from build123d import *

# Parameters (mm, degrees)
BOSS_EXTRUDE1_DEPTH = 70
FILLET1_R           = 10
SKETCH4_R           = 44.565838739
SKETCH4_R_2         = 21.950927137
CUT_EXTRUDE18_DEPTH = 5
SHELL2_START        = 10
SHELL2_DEPTH        = 50
SHELL2_START_2      = -77.141831355
SHELL2_2_OUTLINE_R  = 11.950927137
SHELL2_2_DEPTH      = 25
SKETCH2_R           = 10
CUT_EXTRUDE19_DEPTH = 30
SKETCH10_R          = 7.386058148
CUT_EXTRUDE22_DEPTH = 33
CUT_EXTRUDE23_DEPTH = 131.776604246
SKETCH16_W          = 25
SKETCH16_H          = 5
CUT_EXTRUDE25_DEPTH = 16.122153735
SKETCH17_W          = 25
SKETCH17_H          = 5
CUT_EXTRUDE26_DEPTH = 16.122153735


with BuildPart() as part:
    # Sketch1 → Boss-Extrude1 (new body)
    with BuildSketch(Plane.XY):
        Polygon((-85.15522278, 32.602281584), (85.31682344, 32.602281584), (107.858168645, -0.126017705), (84.012402994, -31.916476628), (-83.600577489, -31.916476628), (-92.141831355, -19.515233034), (-92.141831355, 19.263197625), align=None)
    extrude(amount=BOSS_EXTRUDE1_DEPTH)

    # Fillet1
    fillet1_edges = [part.edges().sort_by_distance(p)[0] for p in [
        (-88.648527067, 25.932739604, 0),
        (-85.15522278, 32.602281584, 35),
        (85.31682344, 32.602281584, 35),
        (107.858168645, -0.126017705, 35),
        (-87.871204422, -25.715854831, 70),
        (84.012402994, -31.916476628, 35),
        (-83.600577489, -31.916476628, 35),
        (-92.141831355, -19.515233034, 35),
        (-92.141831355, 19.263197625, 35),
        (0.205912752, -31.916476628, 70),
        (95.93528582, -16.021247166, 70),
        (96.587496042, 16.23813194, 70),
        (0.08080033, 32.602281584, 70),
        (-88.648527067, 25.932739604, 70),
        (0.08080033, 32.602281584, 0),
        (96.587496042, 16.23813194, 0),
        (95.93528582, -16.021247166, 0),
        (0.205912752, -31.916476628, 0),
        (-92.141831355, -0.126017705, 70),
        (-87.871204422, -25.715854831, 0),
        (-92.141831355, -0.126017705, 0),
    ]]
    fillet(fillet1_edges, radius=FILLET1_R)

    # Sketch4 → Cut-Extrude18 (cut)
    with BuildSketch(Plane(origin=(-62.141831355, 0, 0), x_dir=(0, 0, -1), z_dir=(1, 0, 0))):
        with Locations((-35, -0.126017705)):
            Circle(SKETCH4_R)
        with Locations(Location((-35, -0.126017705, 0), (0, 0, 90))):
            Circle(SKETCH4_R_2, mode=Mode.SUBTRACT)
    extrude(amount=-CUT_EXTRUDE18_DEPTH, mode=Mode.SUBTRACT)

    # Shell2: read off the stored shape, not the designer's step
    # Shell2 outline → Shell2 (cut)
    with BuildSketch(Plane.XY.offset(SHELL2_START)):
        Polygon((-78.345650785, -21.916476628), (-77.141831355, -21.916476628), (-77.141831355, 22.602281584), (-79.104276607, 22.602281584), (-82.141831355, 16.80287299), (-82.141831355, -16.404714454), align=None)
        Polygon((-52.141831355, -21.916476628), (79.012770562, -21.916476628), (95.544357754, 0.122939143), (80.061896735, 22.602281584), (-52.141831355, 22.602281584), align=None)
    extrude(amount=SHELL2_DEPTH, mode=Mode.SUBTRACT)

    # Shell2 2 outline → Shell2 2 (cut)
    with BuildSketch(Plane.YZ.offset(SHELL2_START_2)):
        with Locations((-0.126017705, 35)):
            Circle(SHELL2_2_OUTLINE_R)
    extrude(amount=SHELL2_2_DEPTH, mode=Mode.SUBTRACT)

    # Sketch2 → Cut-Extrude19 (cut)
    with BuildSketch(Plane.ZY.offset(92.141831355)):
        with Locations(Location((35, -0.126017705, 0), (0, 0, 270))):
            Circle(SKETCH2_R)
    extrude(amount=-CUT_EXTRUDE19_DEPTH, mode=Mode.SUBTRACT)

    # Sketch10 → Cut-Extrude22 (cut)
    with BuildSketch(Plane(origin=(7.840565514, -44.466056654, 0), x_dir=(0, 0, 1), z_dir=(0.17364817766693072, -0.984807753012208, 0))):
        with Locations(Location((35.616590305, -27.492158059, 0), (0, 0, 270))):
            Circle(SKETCH10_R)
    extrude(amount=-CUT_EXTRUDE22_DEPTH, mode=Mode.SUBTRACT)

    # Sketch11 → Cut-Extrude23 (cut, through all)
    with BuildSketch(Plane.XY.offset(70)):
        Polygon((25.724647203, 14.602281584), (30.724647203, 14.602281584), (46.292543401, -13.916476628), (41.292543401, -13.916476628), align=None)
        Polygon((21.292543401, -13.916476628), (26.292543401, -13.916476628), (10.724647203, 14.602281584), (5.724647203, 14.602281584), align=None)
        Polygon((45.724647203, 14.602281584), (61.292543401, -13.916476628), (66.292543401, -13.916476628), (50.724647203, 14.602281584), align=None)
    extrude(amount=-CUT_EXTRUDE23_DEPTH, mode=Mode.SUBTRACT)

    # Sketch16 → Cut-Extrude25 (cut)
    with BuildSketch(Plane(origin=(73.09679987, 50.344815805, 0), x_dir=(0, 0, -1), z_dir=(0.8235642198480575, 0.5672230388357482, 0))):
        with Locations((-35, -41.547421266)):
            Rectangle(SKETCH16_W, SKETCH16_H)
    extrude(amount=-CUT_EXTRUDE25_DEPTH, mode=Mode.SUBTRACT)

    # Sketch17 → Cut-Extrude26 (cut)
    with BuildSketch(Plane(origin=(69.08362881, -51.819070211, 0), x_dir=(0, 0, -1), z_dir=(0.7999647115864142, -0.600047048335766, 0))):
        with Locations((-35, 43.629456832)):
            Rectangle(SKETCH17_W, SKETCH17_H)
    extrude(amount=-CUT_EXTRUDE26_DEPTH, mode=Mode.SUBTRACT)


solid = part.part
Could you check a few things on this model? Use its own coordinates, in mm. A direction names the side the tool comes from. Give positions to 0.01 mm unless a question says otherwise; leave off trailing zeros. Loops run counter-clockwise (first coordinate to the right, second up) from the corner with the lowest first, then second, coordinate; pieces in that order, holes last. Notation, with made-up numbers: (45.5, 21) -> (83.5, 21) arc R12 cw to (83.5, 33) -> close; hole circle Ø5 at (87, 82). An arc over 180 degrees is marked (long way). Answer as CSV lines item,"result". Start each with the question number.
(1) If we section it at A-A on z = 64: Count the separate pieces of the cut face and the enclosed holes in it, then the cut area to 3 significant figures.
(2) Which directions (+Z, -Z, +X, -X, +Y, -Y) give clear straight access to the entire face, cutting with the end or side of a thin tool? Please do faces 1 (the cylindrical face through (-72.822, -29.065, 3.007)), 2 (the flat face through (58.62, 0.14, 65.07)), 3 (the flat face through (86.191, 13.703, 34.65)).
(3) I need wall thicknesses on probe 1 along Y at (x, z) = (50, 48); probe 2 along Z at (x, y) = (74, 18); probe 3 along X at (y, z) = (6.5, 10.5). Which ranges of each line are inside material? Lowest first, please.
(4) We'd pull the mould along Z, two halves only. Please class faces 4 (the flat face through (91, -14, 22.5)), 5 (the cylindrical face through (105.544, 0.008, 35.35)), 6 (the flat face through (93, 13, 47.5)), 7 (the cylindrical face through (93.8, 15.26, 3.01)): released by +Z, released by -Z, zero draft, split by the parting line, or undercut.
(5) If we section it at B-B on x = -15: Write out the boundary of the cut face in (y, z), then the cut area to 3 significant figures.
(6) If we section it at C-C on x = 8: Write out the boundary of the cut face in (y, z).
(7) I'm going to push flat-ended pins straight in: pin 1 Ø6 at (y, z) = (8.5, 38.5) entering from +X; pin 2 Ø1.5 at (x, z) = (49, 65) entering from -Y; pin 3 Ø5.5 at (x, z) = (49.5, 6.5) entering from -Y. Where does each tip first touch, or does it pass through?
Computed:
1,separate pieces,"2"
1,enclosed holes,"3"
1,area,"10,900 mm2"
2,face 1,"-Z, +X, -X, -Y"
2,face 2,"+Z, -Z"
2,face 3,"none"
3,probe 1,"y = -31.92 to -21.92, 22.6 to 32.6"
3,probe 2,"z = 0 to 10, 60 to 70"
3,probe 3,"x = -92.14 to -82.14, -77.14 to -67.14, -62.14 to -52.14, 91.15 to 103.29"
4,face 4,"undercut"
4,face 5,"zero draft"
4,face 6,"undercut"
4,face 7,"released by -Z"
5,outline,"(-31.92, 10) arc R10 ccw to (-21.92, 0) -> (22.6, 0) arc R10 ccw to (32.6, 10) -> (32.6, 60) arc R10 ccw to (22.6, 70) -> (-21.92, 70) arc R10 ccw to (-31.92, 60) -> close; hole (-21.92, 10) -> (22.6, 10) -> (22.6, 60) -> (-21.92, 60) -> close"
5,area,"2,200 mm2"
6,outline,"(-31.92, 10) arc R10 ccw to (-21.92, 0) -> (10.43, 0) -> (10.43, 10) -> (-21.92, 10) -> (-21.92, 60) -> (10.43, 60) -> (10.43, 70) -> (-21.92, 70) arc R10 ccw to (-31.92, 60) -> close; (14.6, 0) -> (22.6, 0) arc R10 ccw to (32.6, 10) -> (32.6, 60) arc R10 ccw to (22.6, 70) -> (14.6, 70) -> (14.6, 60) -> (22.6, 60) -> (22.6, 10) -> (14.6, 10) -> close"
7,pin 1,"stops at x = 103.98"
7,pin 2,"stops at y = -30.97"
7,pin 3,"stops at y = -31.89"
